Design review of the part built by this model. Coordinates are the model's own, in mm. Face numbers are marked on the shaded views. A direction names the side the tool comes from. Round coordinates to 2 decimals unless told otherwise and drop trailing zeros. Order: outer loops, then holes, each group sorted by start corner. A loop starts at its lowest first (then second) coordinate and runs counter-clockwise, first axis right, second up.
Autodesk Inventor part; units mm, degrees
ref_plane "YZ Plane" through (0, 0, 0) normal (1, 0, 0) x (0, 1, 0)
ref_plane "XZ Plane" through (0, 0, 0) normal (0, 1, 0) x (-1, 0, 0)
ref_plane "XY Plane" through (0, 0, 0) normal (0, 0, 1) x (1, 0, 0)
ref_plane "Work Plane13" through (0, 3, 0) normal (0, 1, 0) x (1, 0, 0)
sketch "Sketch45" plane through (0, 3, 0) normal (0, 1, 0) x (1, 0, 0)
  line L0 (35, -20) -> (-3, -20)
  line L1 (-3, -20) -> (-3, 20)
  line L2 (-3, 20) -> (35, 20)
  line L3 (35, 20) -> (35, -20)
  point P0 (0, 0)
  dimension "d142" = 38
  dimension "d143" = 40
extrude "Extrusion34" add sketch "Sketch45" along normal blind 30
sketch "Sketch46" plane through (0, 33, 0) normal (0, 1, 0) x (1, 0, 0)
  point P0 (0, 0)
ref_plane "Work Plane11" through (0, 0, 0) normal (0, -1, 0) x (1, 0, 0)
sketch "Sketch47" plane through (0, 0, 0) normal (0, -1, 0) x (1, 0, 0)
  circle A0 centre (16, 0) radius 18
  point P0 (0, 0)
  dimension "d146" = 36
extrude "Extrusion35" cut sketch "Sketch47" against normal blind 30 draft -15
sketch "Sketch48" plane through (0, 33, 0) normal (0, 1, 0) x (1, 0, 0)
  point P0 (0, 0)
sketch "Sketch49" plane through (0, 33, 0) normal (0, 1, 0) x (1, 0, 0)
  circle A0 centre (20, 0) radius 0.5
  point P0 (0, 0)
  dimension "d149" = 1
extrude "Extrusion36" cut sketch "Sketch49" against normal through all
ref_plane "Work Plane7" through (35, 3, -20) normal (0, 0, -1) x (-1, 0, 0)
sketch "Sketch58" plane through (35, 3, -20) normal (0, 0, -1) x (-1, 0, 0)
  line L0 (7, 20) -> (27, 20)
  line L1 (27, 20) -> (27, 5)
  line L2 (27, 5) -> (7, 5)
  line L3 (7, 5) -> (7, 20)
  point P0 (35, -3)
  dimension "d156" = 20
  dimension "d157" = 15
extrude "Extrusion38" cut sketch "Sketch58" against normal blind 15
ref_plane "Work Plane4" through (-3, 3, -20) normal (-1, 0, 0) x (0, 0, 1)
sketch "Sketch59" plane through (-3, 3, -20) normal (-1, 0, 0) x (0, 0, 1)
  line L0 (5, 25) -> (8, 25)
  line L1 (8, 25) -> (8, 5)
  line L2 (8, 5) -> (5, 5)
  line L3 (5, 5) -> (5, 25)
  point P0 (20, -3)
  dimension "d160" = 3
  dimension "d161" = 20
extrude "Extrusion39" cut sketch "Sketch59" against normal blind 35
ref_plane "Work Plane1" through (0, 3, 0) normal (0, 1, 0) x (1, 0, 0)
ref_plane "Work Plane6" through (0, 23, 0) normal (0, 1, 0) x (1, 0, 0)
properties part number "liquid port_v00"
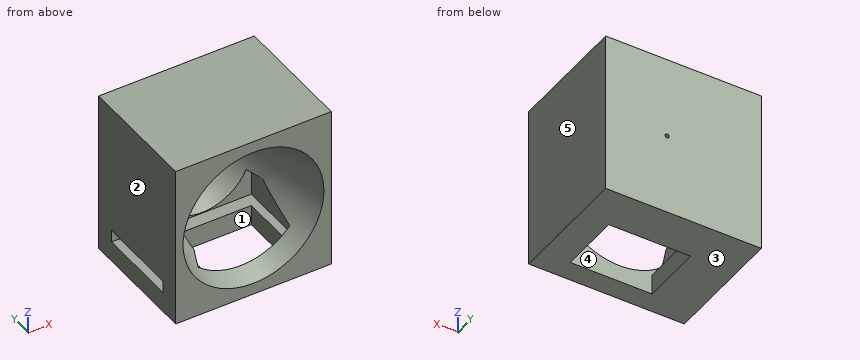
1) To check wall thickness, follow line 1 along X through (y, z) = (30.6, 0); line 2 along Z through (x, y) = (20, 32.35); line 3 along Y through (x, z) = (20.5, -17). State the ranges of each line that lie inside material, in increasing order.
Results:
line 1: x = -3 to 19.5, 20.5 to 35
line 2: z = -20 to -0.5, 0.5 to 20
line 3: y = 3 to 8, 23 to 33
2) Take a section at D-D on y = 5.5. Give the boundary of the cut face in (x, z), plus the area to 3 significant figures.
Results:
outline: (-3, -20) - (35, -20) - (35, 20) - (-3, 20) - close; hole circle Ø33.05 at (16, 0)
area: 662 mm2
3) For the marked faces 1 and 2, list the 3-axis set-ups (+Z, -Z, +X, -X, +Y, -Y) from which the entire face can be reached by the end or side of a thin tool; tool diameter is ignored.
Results:
face 1: -Z
face 2: +Z, -Z, -X, +Y, -Y
4) Clearance check with flat-ended pins moving along their axes: P1, Ø0.9, axis at y = 18.5, z = -14, coming from the -X side; P2, Ø16, axis at x = 16.5, z = 0.5, coming from the -Y side; P3, Ø2, axis at x = 17.5, y = 21, coming from the -Z side (3 decimals). State where each tip first meets the part, or that it passes through.
Results:
P1: stops at x = 32
P2: stops at y = 30
P3: stops at z = 11.975
5) The part is to be moulded in two halves that separate along Z. For the marked faces 3, 4 and 5, say which applies: released by +Z, released by -Z, zero draft, split by the parting line, or undercut.
Results:
face 3: released by -Z
face 4: undercut
face 5: zero draft
6) Take a section at A-A on z = -18. Give the boundary of the cut face in (x, y).
Results:
outline: (-3, 3) - (35, 3) - (35, 33) - (-3, 33) - close; hole (8, 8) - (28, 8) - (28, 23) - (8, 23) - close
7) Take a section at B-B on y = 24. Give the boundary of the cut face in (x, z), plus the area to 3 significant figures.
Results:
outline: (-3, -20) - (35, -20) - (35, 20) - (-3, 20) - (-3, -12) - (32, -12) - (32, -15) - (-3, -15) - close; hole circle Ø23.14 at (16, 0)
area: 995 mm2
8) Take a section at C-C on x = 16. Give the boundary of the cut face in (y, z), plus the area to 3 significant figures.
Results:
outline: (3, -20) - (8, -20) - (8, -15.86) - (3, -17.2) - close; (3, 17.2) - (30, 9.96) - (30, -9.96) - (23, -11.84) - (23, -12) - (28, -12) - (28, -15) - (23, -15) - (23, -20) - (33, -20) - (33, 20) - (3, 20) - close
area: 359 mm2
